Autodesk Inventor part; units mm, degrees
ref_plane "YZ Plane" through (0, 0, 0) normal (1, 0, 0) x (0, 1, 0)
ref_plane "XZ Plane" through (0, 0, 0) normal (0, 1, 0) x (-1, 0, 0)
ref_plane "XY Plane" through (0, 0, 0) normal (0, 0, 1) x (1, 0, 0)
sketch "Sketch1" plane through (0, 0, 0) normal (0, 0, 1) x (1, 0, 0)
  line L0 (-24, -18.5) -> (24, -18.5)
  line L1 (24, -18.5) -> (24, 18.5)
  line L2 (24, 18.5) -> (-24, 18.5)
  line L3 (-24, 18.5) -> (-24, -18.5)
  line L4 (-24, -18.5) -> (24, 18.5) construction
  line L5 (24, -18.5) -> (-24, 18.5) construction
  point P0 (0, 0)
  dimension "d0" = 48
  dimension "d1" = 37
extrude "Extrusion1" add sketch "Sketch1" along normal mid plane 40
chamfer "Chamfer1" distance 5 angle 45 2 edges at (24, -18.5, 0) (-24, -18.5, 0)
sketch "Sketch2" plane through (0, 0, 20) normal (0, 0, 1) x (1, 0, 0)
  line L0 (24, 18.5) -> (-24, 18.5)
  point P0 (0, 0)
  point P1 (0, -0.5)
  point P2 (0, 18.5)
  dimension "d7" = 19
hole "Hole1" at (0, -0.5, 20) direction (0, 0, -1) diameter 30.5 end through all
chamfer "Chamfer2" distance 0.5 angle 45 2 edges at (0, 14.75, 20) (0, 14.75, -20)
sketch "Sketch3" plane through (-24, 18.5, 20) normal (0, 1, 0) x (1, 0, 0)
  line L0 (44, 7.5) -> (4, 7.5)
  line L1 (4, 7.5) -> (4, 32.5)
  line L2 (4, 32.5) -> (44, 32.5)
  line L3 (44, 32.5) -> (44, 7.5)
  line L4 (44, 7.5) -> (4, 32.5) construction
  line L5 (4, 7.5) -> (44, 32.5) construction
  point P0 (24, 20)
  dimension "d18" = 25
  dimension "d19" = 40
hole "Hole2" at (-20, 18.5, -12.5) at (-20, 18.5, 12.5) at (20, 18.5, -12.5) at (20, 18.5, 12.5) direction (0, -1, 0) diameter 3.242 depth 12 tip angle 118
sketch "Sketch4" plane through (0, 0, 20) normal (0, 0, 1) x (1, 0, 0)
  circle A0 centre (0, -0.5) radius 20 construction
  circle A1 centre (0, -0.5) radius 15.25
  point P0 (0, 0)
  point P1 (-17.3205, 9.5)
  point P2 (-17.3205, -10.5)
  point P3 (17.3205, -10.5)
  point P4 (17.3205, 9.5)
  dimension "d27" = 20
  dimension "d28" = 40
hole "Hole4" at (-17.3205, 9.5, 20) at (-17.3205, -10.5, 20) at (17.3205, -10.5, 20) at (17.3205, 9.5, 20) direction (0, 0, -1) diameter 3.242 depth 10 tip angle 118
properties part number "Ballnut_Support"
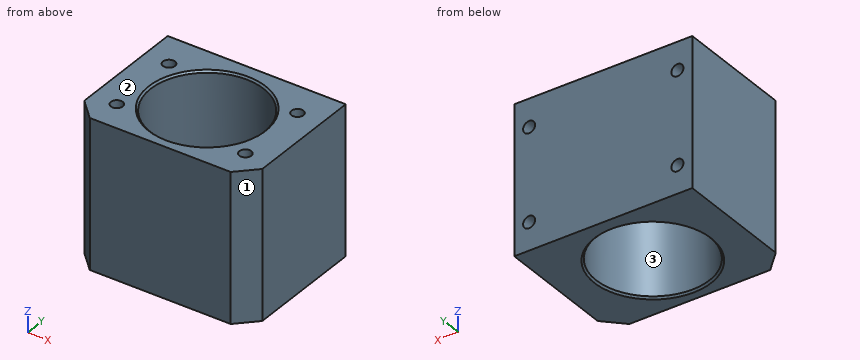
The listing builds one solid part. Answer for the finished solid, in the listing's coordinates (mm). Face numbers are marked on the shaded views. Coordinates: 2 decimals unless noted, no trailing zeros. Write each loop counter-clockwise with the first axis right and the second up, starting at its lowest first coordinate (ties: lowest second). Pieces come first, ordered by that corner, then holes. Notation, with made-up numbers: (0.25, 30) - (32.25, 30) arc R24 cw to (32.25, 45) - close; hole circle Ø5 at (26.5, -1). An arc over 180 degrees is marked (long way). Return JSON: item names as keys, results as strings. Group by question number.
Q1. The part is cut by section B-B on z = -4.5. Write down the section's boundary in (x, y).
Q2. Find the intervals of material crossed by line 1 along Z through (x, y) = (-20, 15.5); line 2 along X through (y, z) = (15, -12.5); line 3 along X through (y, z) = (13, 12), in increasing order. Write a range as [from, to].
Q3. For a pull along Y with two mould halves and no side action, classify the marked faces 1, 2 and 3 as +Y half, -Y half, draft (parallel to the pull), parting line (faces both ways), or undercut.
Q4. Flat-ended cylindrical pins translate along their axes: pin 1 Ø3 at (x, y) = (17.32, -10.5) entering from +Z; pin 2 Ø1.9 at (x, z) = (-20, 12.5) entering from +Y; pin 3 Ø2.5 at (x, z) = (-20, -12.5) entering from +Y. Find the tip coordinate at first contact, or state that the pin passes through.
Q5. The part is cut by section A-A on x = 0. Write down the section's boundary in (y, z).
Evaluation:
{
 "1": {"outline": "(-24, -13.5) - (-19, -18.5) - (19, -18.5) - (24, -13.5) - (24, 18.5) - (-24, 18.5) - close; hole circle Ø30.5 at (0, -0.5)"},
 "2": {"line 1": "z = [-20, -14.12], [-10.88, 10.88], [14.12, 20]", "line 2": "x = [-24, -21.62], [-18.38, 18.38], [21.62, 24]", "line 3": "x = [-24, -21.54], [-18.46, -7.09], [7.09, 18.46], [21.54, 24]"},
 "3": {"face 1": "-Y half", "face 2": "draft", "face 3": "undercut"},
 "4": {"pin 1": "stops at z = 9.93", "pin 2": "stops at y = 6.1", "pin 3": "stops at y = 6.28"},
 "5": {"outline": "(-18.5, -20) - (-16.25, -20) - (-15.75, -19.5) - (-15.75, 19.5) - (-16.25, 20) - (-18.5, 20) - close; (14.75, -19.5) - (15.25, -20) - (18.5, -20) - (18.5, 20) - (15.25, 20) - (14.75, 19.5) - close"}
}
